```python
from build123d import *

# Parameters (mm, degrees)
SKETCH1_R           = 3.175
BOSS_EXTRUDE1_DEPTH = 44.45
SKETCH3_R           = 2.6416
BOSS_EXTRUDE2_DEPTH = 0.762
SKETCH4_R           = 3.175
BOSS_EXTRUDE3_DEPTH = 3.175
BOSS_EXTRUDE4_START = 0.762
SKETCH5_R           = 2.6416
BOSS_EXTRUDE4_DEPTH = 0.762
BOSS_EXTRUDE5_START = 3.175
SKETCH6_R           = 3.175
BOSS_EXTRUDE5_DEPTH = 3.175


with BuildPart() as part:
    # Sketch1 → Boss-Extrude1 (new body)
    with BuildSketch(Plane(origin=(0, 0, 0), x_dir=(1, 0, 0), z_dir=(0, 1, 0))):
        with Locations(Location((0, 0, 0), (0, 0, 270))):
            Circle(SKETCH1_R)
    extrude(amount=BOSS_EXTRUDE1_DEPTH)

    # Sketch3 → Boss-Extrude2 (add)
    with BuildSketch(Plane(origin=(0, 44.45, 0), x_dir=(1, 0, 0), z_dir=(0, 1, 0))):
        with Locations(Location((0, 0, 0), (0, 0, 90))):
            Circle(SKETCH3_R)
    extrude(amount=BOSS_EXTRUDE2_DEPTH)

    # Sketch4 → Boss-Extrude3 (add)
    with BuildSketch(Plane(origin=(0, 45.212, 0), x_dir=(1, 0, 0), z_dir=(0, 1, 0))):
        with Locations(Location((0, 0, 0), (0, 0, 270))):
            Circle(SKETCH4_R)
    extrude(amount=BOSS_EXTRUDE3_DEPTH)

    # Sketch5 → Boss-Extrude4 (add)
    with BuildSketch(Plane.XZ.offset(BOSS_EXTRUDE4_START)):
        with Locations(Location((0, 0, 0), (0, 0, 270))):
            Circle(SKETCH5_R)
    extrude(amount=-BOSS_EXTRUDE4_DEPTH)

    # Sketch6 → Boss-Extrude5 (add)
    with BuildSketch(Plane.XZ.offset(0.762).offset(BOSS_EXTRUDE5_START)):
        with Locations(Location((0, 0, 0), (0, 0, 90))):
            Circle(SKETCH6_R)
    extrude(amount=-BOSS_EXTRUDE5_DEPTH)


solid = part.part
```
CAD build for the part. Positions are in the model's coordinates, mm. A direction names the side the tool comes from. Coordinates: 2 decimals unless noted, no trailing zeros. Loops run counter-clockwise (first coordinate to the right, second up) from the corner with the lowest first, then second, coordinate; pieces in that order, holes last. Notation, with made-up numbers: (26.5, -17) - (56.5, -17) arc R22 cw to (56.5, 8) - close; hole circle Ø10 at (36.5, -38.5). An arc over 180 degrees is marked (long way). Use CSV: the item, a comma, the result in double quotes. Start each with the question number.
Q1. Two-plate mould, pull along Y, no slides. Class faces 1 (the cylindrical face through (1.6, 44.8, 2.1)), 2 (the flat face through (-2, -0.762, -2)), 3 (the cylindrical face through (-1.93, 46.78, -2.52)), 4 (the flat face through (0, -3.937, 0)): +Y half, -Y half, draft (parallel to the pull), parting line (faces both ways), or undercut.
Q2. 3-axis set-ups, long thin cutter, end or side, ignore diameter. For faces 5 (the flat face through (2, 0, -2)), 6 (the flat face through (0, 48.387, 0)): which of +Z, -Z, +X, -X, +Y, -Y reach the whole face in a straight line?
Q3. Cut at B-B, the plane y = 4.5. List the corners of the cut face in (x, z) (3 decimals).
Q4. Probe probe 1 along Y at (x, z) = (-2.25, 1.5); probe 2 along Z at (x, y) = (-0.25, 25); probe 3 along Z at (x, y) = (1.75, 0.5). List the from-to ranges inside material, lowest first. Write a range as from..to.
Q5. Cut at C-C, the plane x = 2. List the corners of the cut face in (y, z).
Q6. Cut at A-A, the plane x = -1.5. List the corners of the cut face in (y, z), then the cut area to 3 significant figures.
Q7. Drop flat-ended pins along their axis: P1, Ø3, axis at x = -1.5, y = 39, coming from the -Z side (3 decimals); P2, Ø2, axis at y = 20.5, z = 1.5, coming from the -X side. Give the stop position or say it passes through.
Here are the results:
1,face 1,"undercut"
1,face 2,"undercut"
1,face 3,"draft"
1,face 4,"-Y half"
2,face 5,"none"
2,face 6,"+Z, -Z, +X, -X, +Y"
3,outline,"circle Ø6.35 at (0, 0)"
4,probe 1,"-3.94..-0.76, 0..44.45, 45.21..48.39"
4,probe 2,"-3.17..3.17"
4,probe 3,"-2.65..2.65"
5,outline,"(-3.94, -2.47) - (-0.76, -2.47) - (-0.76, -1.73) - (0, -1.73) - (0, -2.47) - (44.45, -2.47) - (44.45, -1.73) - (45.21, -1.73) - (45.21, -2.47) - (48.39, -2.47) - (48.39, 2.47) - (45.21, 2.47) - (45.21, 1.73) - (44.45, 1.73) - (44.45, 2.47) - (0, 2.47) - (0, 1.73) - (-0.76, 1.73) - (-0.76, 2.47) - (-3.94, 2.47) - close"
6,outline,"(-3.94, -2.8) - (-0.76, -2.8) - (-0.76, -2.17) - (0, -2.17) - (0, -2.8) - (44.45, -2.8) - (44.45, -2.17) - (45.21, -2.17) - (45.21, -2.8) - (48.39, -2.8) - (48.39, 2.8) - (45.21, 2.8) - (45.21, 2.17) - (44.45, 2.17) - (44.45, 2.8) - (0, 2.8) - (0, 2.17) - (-0.76, 2.17) - (-0.76, 2.8) - (-3.94, 2.8) - close"
6,area,"291 mm2"
7,P1,"z = -3.175"
7,P2,"x = -3.14"
